```python
from build123d import *

# Parameters (mm, degrees)
SKETCH2_W                = 12
SKETCH2_H                = 120
BOSS_EXTRUDE1_DEPTH      = 10
FILLET1_R                = 5
CUT_EXTRUDE1_DEPTH       = 3
CUT_EXTRUDE2_START       = 7
SKETCH3_2_W              = 12
SKETCH3_2_H              = 9
CUT_EXTRUDE2_DEPTH       = 3
CUT_EXTRUDE4_START       = -4
CUT_EXTRUDE4_DEPTH       = 66.12282716
SKETCH7_R                = 1.5
CUT_EXTRUDE5_DEPTH       = 61.704200843
BOSS_EXTRUDE2_DEPTH      = 7
BOSS_EXTRUDE2_DEPTH_BACK = 7
SKETCH9_W                = 15
SKETCH9_H                = 80
FILLET3_R                = 7


with BuildPart() as part:
    # Sketch2 → Boss-Extrude1 (new body)
    with BuildSketch(Plane.XY):
        Rectangle(SKETCH2_W, SKETCH2_H)
    extrude(amount=BOSS_EXTRUDE1_DEPTH)

    # Fillet1
    fillet1_edges = [part.edges().sort_by_distance(p)[0] for p in [
        (-6, 0, 0),
        (6, 0, 0),
        (6, 0, 10),
        (-6, 0, 10),
    ]]
    fillet(fillet1_edges, radius=FILLET1_R - 0.0001)  # a hair under: the kernel refuses the full size

    # Sketch3 → Cut-Extrude1 (cut)
    with BuildSketch(Plane.XY):
        with BuildLine():
            Line((-6, -51), (-4.5, -55.5))
            ThreePointArc((-4.5, -55.5), (0, -60), (4.5, -55.5))
            Line((4.5, -55.5), (6, -51))
            Line((6, -51), (-6, -51))
        make_face()
        with BuildLine():
            Line((0, -60), (6, -60))
            Line((6, -60), (6, -51))
            Line((6, -51), (4.5, -55.5))
            ThreePointArc((4.5, -55.5), (3.181980515, -58.681980515), (0, -60))
        make_face()
        with BuildLine():
            Line((-6, -60), (0, -60))
            ThreePointArc((0, -60), (-3.181980515, -58.681980515), (-4.5, -55.5))
            Line((-4.5, -55.5), (-6, -51))
            Line((-6, -51), (-6, -60))
        make_face()
    cut_extrude1 = extrude(amount=CUT_EXTRUDE1_DEPTH, mode=Mode.SUBTRACT)

    # Sketch3<2> → Cut-Extrude2 (cut)
    with BuildSketch(Plane.XY.offset(CUT_EXTRUDE2_START)):
        with Locations((0, -55.5)):
            Rectangle(SKETCH3_2_W, SKETCH3_2_H)
    cut_extrude2 = extrude(amount=CUT_EXTRUDE2_DEPTH, mode=Mode.SUBTRACT)

    # Mirror1: Cut-Extrude1, Cut-Extrude2 across plane
    add(cut_extrude1.mirror(Plane.ZX), mode=Mode.SUBTRACT)
    add(cut_extrude2.mirror(Plane.ZX), mode=Mode.SUBTRACT)

    # Sketch3<4> → Cut-Extrude4 (cut)
    with BuildSketch(Plane.XY.offset(CUT_EXTRUDE4_START)):
        with BuildLine():
            Line((0, -60), (6, -60))
            Line((6, -60), (6, -51))
            Line((6, -51), (4.5, -55.5))
            ThreePointArc((4.5, -55.5), (3.181980515, -58.681980515), (0, -60))
        make_face()
        with BuildLine():
            Line((-6, -60), (0, -60))
            ThreePointArc((0, -60), (-3.181980515, -58.681980515), (-4.5, -55.5))
            Line((-4.5, -55.5), (-6, -51))
            Line((-6, -51), (-6, -60))
        make_face()
    cut_extrude4 = extrude(amount=CUT_EXTRUDE4_DEPTH, mode=Mode.SUBTRACT)

    # Sketch7 → Cut-Extrude5 (cut, through all)
    with BuildSketch(Plane(origin=(0, 0, 3), x_dir=(-1, 0, 0), z_dir=(0, 0, -1))):
        with Locations((0, -55.5)):
            Circle(SKETCH7_R)
    cut_extrude5 = extrude(amount=-CUT_EXTRUDE5_DEPTH, mode=Mode.SUBTRACT)

    # Mirror3: Cut-Extrude5 across plane
    add(cut_extrude5.mirror(Plane.ZX), mode=Mode.SUBTRACT)

    # Mirror4: Cut-Extrude4 across plane
    add(cut_extrude4.mirror(Plane.ZX), mode=Mode.SUBTRACT)

    # Sketch9 → Boss-Extrude2 (add, two sides: drawn at the far end of the back side and taken through both)
    with BuildSketch(Plane.XY.offset(5).offset(-BOSS_EXTRUDE2_DEPTH_BACK)):
        Rectangle(SKETCH9_W, SKETCH9_H)
    extrude(amount=BOSS_EXTRUDE2_DEPTH + BOSS_EXTRUDE2_DEPTH_BACK)

    # Fillet3
    fillet3_edges = [part.edges().sort_by_distance(p)[0] for p in [
        (-7.5, 0, 12),
        (7.5, 0, 12),
        (7.5, 0, -2),
        (-7.5, 0, -2),
    ]]
    fillet(fillet3_edges, radius=FILLET3_R - 0.0001)  # a hair under: the kernel refuses the full size


solid = part.part
```
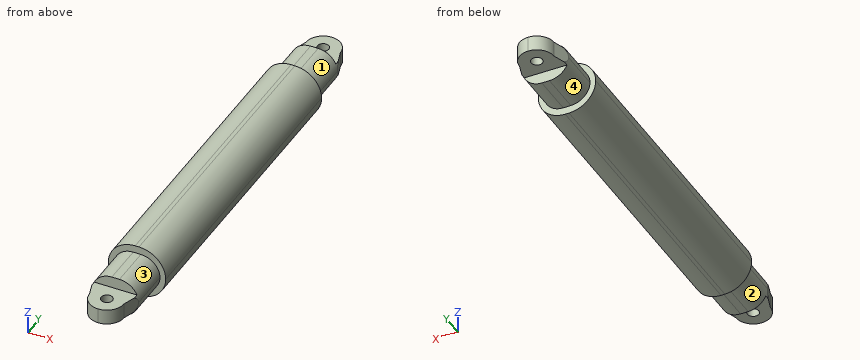
Verification items for the finished model (mm, model axes). Face numbers are marked on the shaded views. A direction names the side the tool comes from. Round coordinates to 2 decimals unless told otherwise and drop trailing zeros. Order: outer loops, then holes, each group sorted by start corner. A loop starts at its lowest first (then second) coordinate and runs counter-clockwise, first axis right, second up.
1) Cross-section at B-B, the plane x = -2.5. Record the cut outline in (y, z), plus the area to 3 significant figures.
Geometry says:
outline: (-59.24, 3) - (-51, 3) - (-51, 0.23) - (-40, 0.23) - (-40, -1.71) - (40, -1.71) - (40, 0.23) - (51, 0.23) - (51, 3) - (59.24, 3) - (59.24, 7) - (51, 7) - (51, 9.77) - (40, 9.77) - (40, 11.71) - (-40, 11.71) - (-40, 9.77) - (-51, 9.77) - (-51, 7) - (-59.24, 7) - close
area: 1,350 mm2
2) Tool access check on the marked faces 1, 2, 3 and 4. Record the directions out of +Z, -Z, +X, -X, +Y, -Y that give a thin tool (end or side, any length) a straight path to the whole face; none if there is none.
Geometry says:
face 1: +Z, +X, +Y
face 2: -Z, -X, -Y
face 3: +Z, +X, -Y
face 4: -Z, -X, +Y
3) Material ranges on line 1 (Y direction, x = 0, z = 4); line 2 (X direction, y = 55.5, z = 4.7); line 3 (Y direction, x = 5.25, z = 8.75), recorded low to high.
Geometry says:
line 1: y = -60 to -57, -54 to 54, 57 to 60
line 2: x = -4.5 to -1.5, 1.5 to 4.5
line 3: y = -40 to 40
4) Cross-section at D-D, the plane x = 3. Record the cut outline in (y, z).
Geometry says:
outline: (-58.85, 3) - (-51, 3) - (-51, 0.42) - (-40, 0.42) - (-40, -1.54) - (40, -1.54) - (40, 0.42) - (51, 0.42) - (51, 3) - (58.85, 3) - (58.85, 7) - (51, 7) - (51, 9.58) - (40, 9.58) - (40, 11.54) - (-40, 11.54) - (-40, 9.58) - (-51, 9.58) - (-51, 7) - (-58.85, 7) - close
5) Depth check by flat-ended pin: pin 1 (3 mm diameter, centred on x = -2.5, y = -29.5, fed in from +Z); pin 2 (3.5 mm diameter, centred on x = 0, y = -55.5, fed in from +Z); pin 3 (1.5 mm diameter, centred on x = -2.5, z = 8.5, fed in from -Y); pin 4 (1.8 mm diameter, centred on x = 0, y = 55.5, fed in from +Z). Enter the tip coordinate at first touch or a pass-through.
Geometry says:
pin 1: stops at z = 11.98
pin 2: stops at z = 7
pin 3: stops at y = -51
pin 4: passes through
